Part model, mm, in its own coordinate system. Round coordinates to 2 decimals unless told otherwise and drop trailing zeros. Loops run counter-clockwise (first coordinate to the right, second up) from the corner with the lowest first, then second, coordinate; pieces in that order, holes last. Notation, with made-up numbers: (8, 72.5) -> (44, 72.5) arc R29 ccw to (44, 97.5) -> close; hole circle Ø5 at (53.25, 37). An arc over 180 degrees is marked (long way). Answer as a JSON object with one key per item and string values. Group by question number.
from build123d import *

# Parameters (mm, degrees)
BOSS_EXTRUDE1_DEPTH = 152.4


with BuildPart() as part:
    # Sketch2 → Boss-Extrude1 (new, symmetric)
    with BuildSketch(Plane.XY):
        with BuildLine():
            Line((-12.7, -12.7), (12.7, -12.7))
            Line((12.7, -12.7), (12.7, 12.7))
            Line((12.7, 12.7), (11.1125, 12.7))
            ThreePointArc((11.1125, 12.7), (9.989967985, 12.235032015), (9.525, 11.1125))
            Line((9.525, 11.1125), (9.525, -6.35))
            ThreePointArc((9.525, -6.35), (8.59506403, -8.59506403), (6.35, -9.525))
            Line((6.35, -9.525), (-11.1125, -9.525))
            ThreePointArc((-11.1125, -9.525), (-12.235032015, -9.989967985), (-12.7, -11.1125))
            Line((-12.7, -11.1125), (-12.7, -12.7))
        make_face()
    extrude(amount=BOSS_EXTRUDE1_DEPTH, both=True)


solid = part.part
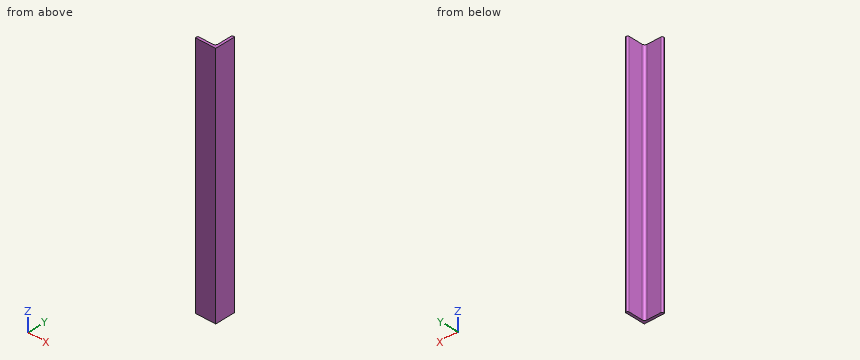
Item 1: Band-saw the part on C-C, the plane x = -4.25. List the corners of the cut face in (y, z) (3 decimals), plus the area to 3 significant figures.
Item 2: Band-saw the part on B-B, the plane y = 2. List the corners of the cut face in (x, z) (3 decimals).
Item 3: Drill centre lines: line 1 (Y direction, x = -4, z = 123) (3 decimals); line 2 (X direction, y = 4.25, z = -118) (3 decimals); line 3 (X direction, y = -11, z = -61.5). Where is each one in solid material? Low to high.
Item 4: Drop flat-ended pins along their axis: pin 1 Ø8.5 at (x, z) = (-3, -13.5) entering from +Y (3 decimals); pin 2 Ø14 at (y, z) = (3, -11) entering from -X (3 decimals); pin 3 Ø10 at (x, y) = (6, 6.5) entering from -Z. Give the stop position or say it passes through.
Entries:
{
 "1": {"outline": "(-12.7, -152.4) -> (-9.525, -152.4) -> (-9.525, 152.4) -> (-12.7, 152.4) -> close", "area": "968 mm²"},
 "2": {"outline": "(9.525, -152.4) -> (12.7, -152.4) -> (12.7, 152.4) -> (9.525, 152.4) -> close"},
 "3": {"line 1": "-12.7 to -9.525", "line 2": "9.525 to 12.7", "line 3": "-12.7 to 12.7"},
 "4": {"pin 1": "y = -9.525", "pin 2": "x = 9.525", "pin 3": "z = -152.4"}
}
